from build123d import *

# Parameters (mm, degrees)
PAD011_DEPTH = 7.5
SKETCH014_W  = 15
SKETCH014_H  = 29.2426
PAD012_DEPTH = 1.2
PAD013_DEPTH = 1.2


with BuildPart() as part:
    # Sketch015 → Pad011 (new body, symmetric)
    with BuildSketch(Plane.YZ):
        with BuildLine():
            Line((-11.85, 3.8), (-13.15, 3.8))
            Line((-13.15, 3.8), (-7.4, 1.9))
            Line((-7.4, 1.9), (-13.15, 0))
            ThreePointArc((-13.15, 0), (-13.279654, -0.257625), (-13.022029, -0.387279))
            Line((-13.022029, -0.387279), (-6.1, 1.9))
            Line((-6.1, 1.9), (-11.85, 3.8))
        make_face()
    pad011 = extrude(amount=PAD011_DEPTH, both=True)

    # Sketch014 (on DatumPlane) → Pad012 (join)
    with BuildSketch(Plane.XY.offset(3.8)):
        Rectangle(SKETCH014_W, SKETCH014_H)
    extrude(amount=PAD012_DEPTH)

    # Mirrored002: Pad011 across Sketch015 V_Axis
    add(pad011.mirror(Plane(origin=(0, 0, 0), x_dir=(1, 0, 0), z_dir=(0, 1, 0))))

    # Sketch018 → Pad013 (join)
    with BuildSketch(Plane.XY.offset(5)):
        Polygon((4, 0), (0, 4), (-4, 0), (0, -4), align=None)
    extrude(amount=PAD013_DEPTH)


solid = part.part
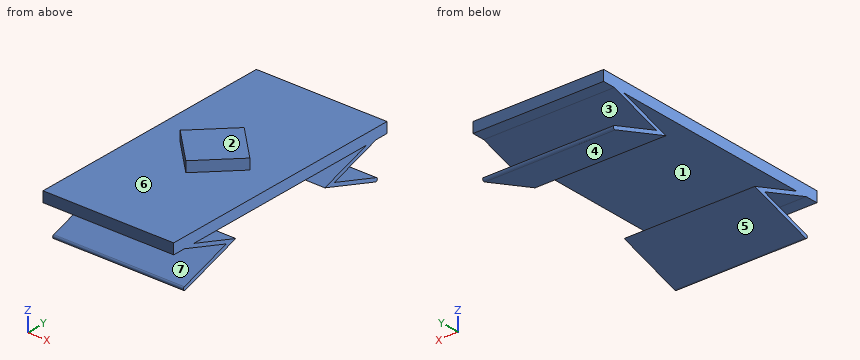
Work out the finished part from the listing and answer in its coordinate system (mm). Face numbers are marked on the shaded views. A direction names the side the tool comes from. Round coordinates to 2 decimals unless told otherwise and drop trailing zeros. Order: outer loops, then holes, each group sorted by start corner. A loop starts at its lowest first (then second) coordinate and runs counter-clockwise, first axis right, second up. Notation, with made-up numbers: M -30,87.5 L -24,87.5 A24 cw -24,110.5 Z; hole C -25.75,84.25 d6. An arc over 180 degrees is marked long. One line per item, written item: value.
Q1. Straight lines are drawn through the part: line 1 (Z direction, x = 6.25, y = 8.5); line 2 (Z direction, x = -0.25, y = 9); line 3 (Z direction, x = 2.25, y = -4.5). For each, find the intervals that lie inside material, in ascending order.
Derived:
line 1: 1.11 to 1.54, 2.26 to 2.69, 3.8 to 5
line 2: 0.94 to 1.37, 2.43 to 2.86, 3.8 to 5
line 3: 3.8 to 5
Q2. For the marked faces 1, 2, 3 and 4, determine the directions among +Z, -Z, +X, -X, +Y, -Y from which every point of the face is accessible in a straight line to the end or side of a thin tool.
Derived:
face 1: +X, -X
face 2: +Z, +X, -X, +Y, -Y
face 3: +X, -X, +Y
face 4: -Z, +X, -X
Q3. Find section C-C on y = -9.25. Write down the section's boundary in (x, z).
Derived:
outline: M -7.5,0.86 L 7.5,0.86 L 7.5,1.29 L -7.5,1.29 Z; M -7.5,2.51 L 7.5,2.51 L 7.5,2.94 L -7.5,2.94 Z; M -7.5,3.8 L 7.5,3.8 L 7.5,5 L -7.5,5 Z
Q4. Find section B-B on x = -0.5. Write down the section's boundary in (y, z).
Derived:
outline: M -14.62,3.8 L -13.15,3.8 L -7.4,1.9 L -13.15,0 A0.2 ccw -13.02,-0.39 L -6.1,1.9 L -11.85,3.8 L 11.85,3.8 L 6.1,1.9 L 13.02,-0.39 A0.2 ccw 13.15,0 L 7.4,1.9 L 13.15,3.8 L 14.62,3.8 L 14.62,5 L 3.5,5 L 3.5,6.2 L -3.5,6.2 L -3.5,5 L -14.62,5 Z
Q5. Flat-ended cylindrical pins translate along their axes: pin 1 (1 mm diameter, centred on x = -2.5, y = -9, fed in from -Z); pin 2 (2 mm diameter, centred on x = -5, y = -11, fed in from +Z); pin 3 (0.7 mm diameter, centred on x = -0.5, y = 13.5, fed in from -Z). Find the tip coordinate at first contact, or state that the pin passes through.
Derived:
pin 1: z = 0.78
pin 2: z = 5
pin 3: z = -0.39
Q6. Determine the mould class of the marked faces 5, 6 and 7 for opening direction Z: released by +Z, released by -Z, zero draft, split by the parting line, or undercut.
Derived:
face 5: released by -Z
face 6: released by +Z
face 7: undercut
Q7. Find section A-A on z = 1.25. Write down the section's boundary in (x, y), then the cut area to 3 significant figures.
Derived:
outline: M -7.5,-9.37 L 7.5,-9.37 L 7.5,-8.07 L -7.5,-8.07 Z; M -7.5,8.07 L 7.5,8.07 L 7.5,9.37 L -7.5,9.37 Z
area: 39.0 mm²
Q8. Find section D-D on y = 1.25. Write down the section's boundary in (x, z).
Derived:
outline: M -7.5,3.8 L 7.5,3.8 L 7.5,5 L 2.75,5 L 2.75,6.2 L -2.75,6.2 L -2.75,5 L -7.5,5 Z
